Here's how the part is built. I have some questions about the finished solid (model axes, mm). A direction names the side the tool comes from. Round coordinates to 2 decimals unless told otherwise and drop trailing zeros. Write each loop counter-clockwise with the first axis right and the second up, starting at its lowest first coordinate (ties: lowest second). Pieces come first, ordered by that corner, then holes. Notation, with made-up numbers: (-37, -35.5) - (6, -35.5) arc R27 cw to (6, 2.5) - close; hole circle Ø8 at (79.5, 62.25). An arc over 180 degrees is marked (long way). One line per question, with ' | ' between items. Start each with the question number.
(1) Will these pins go through, and if not, where does the flat tip stop? pin 1 (1.5 mm diameter, centred on y = 41, z = 5, fed in from -X); pin 2 (5 mm diameter, centred on x = -3.5, y = 14.5, fed in from -Z); pin 3 (3 mm diameter, centred on y = 60, z = 5.5, fed in from +X).
(2) For faces 1 (the flat face through (-9.1, 33, 3)), 2 (the flat face through (6.1, 35, 3)), 3 (the flat face through (9.1, 34, 3)), which set-ups out of +Z, -Z, +X, -X, +Y, -Y let a thin tool reach every point of the face, with its end or its side?
(3) If I drill on L1, parallel to X at y = 9, z = 1.85; L2, parallel to Z at x = -13, y = 71; L3, parallel to Y at x = -13, z = 5.4, over which ranges is the centre line in solid material (lowest first)?
(4) Imagine slicing it at B-B (z = 3). Write out the boundary of the cut face in (x, y), plus the area to 3 significant figures.
(5) Imagine slicing it at A-A (y = 46.5). Write out the boundary of the cut face in (x, z).
(6) Imagine slicing it at C-C (x = 13.1). Write out the boundary of the cut face in (y, z).
(7) Imagine slicing it at D-D (x = -4). Write out the boundary of the cut face in (y, z).
(8) Thinking about a two-plate mould opening in Z: for faces 4 (the cylindrical face through (11.884, 71.479, 4.115)), 5 (the flat face through (17.1, 72, 3)), 6 (the flat face through (-6.3, 34.2, 6)), 7 (the flat face through (-6.3, 34.2, 0)), which applies, pulls with the +Z half, pulls with the -Z half, needs draft (parallel to the pull), parting line crosses it, or undercut?
from build123d import *

# Parameters (mm, degrees)
BOSS_EXTRUDE5_DEPTH = 6
SKETCH7_R           = 1.65
CUT_EXTRUDE2_DEPTH  = 3
FILLET1_R           = 1
FILLET2_R           = 1.5


with BuildPart() as part:
    # Sketch6 → Boss-Extrude5 (new body)
    with BuildSketch(Plane.XY):
        Polygon((-6.1, 0), (6.1, 0), (6.1, 73), (17.1, 73), (17.1, 70), (9.1, 70), (9.1, -5), (-9.1, -5), (-9.1, 70), (-17.1, 70), (-17.1, 73), (-6.1, 73), align=None)
    extrude(amount=BOSS_EXTRUDE5_DEPTH)

    # Sketch7 → Cut-Extrude2 (cut)
    with BuildSketch(Plane.XZ.offset(-70)):
        with Locations((-13.1, 3)):
            Circle(SKETCH7_R)
        with Locations((13.1, 3)):
            Circle(SKETCH7_R)
    extrude(amount=-CUT_EXTRUDE2_DEPTH, mode=Mode.SUBTRACT)

    # Fillet1
    fillet1_edges = [part.edges().sort_by_distance(p)[0] for p in [
        (6.1, 73, 3),
        (-6.1, 73, 3),
    ]]
    fillet(fillet1_edges, radius=FILLET1_R)

    # Fillet2
    fillet2_edges = [part.edges().sort_by_distance(p)[0] for p in [
        (9.1, -5, 3),
        (-9.1, -5, 3),
    ]]
    fillet(fillet2_edges, radius=FILLET2_R)


solid = part.part
Check sheet entries:
1) pin 1: x = -9.1 | pin 2: through | pin 3: x = 9.1
2) face 1: +Z, -Z, -X, -Y | face 2: +Z, -Z, +Y | face 3: +Z, -Z, +X, -Y
3) L1: -9.1 to -6.1, 6.1 to 9.1 | L2: 0 to 1.35, 4.65 to 6 | L3: 70 to 73
4) outline: (-17.1, 70) - (-14.75, 70) - (-14.75, 73) - (-17.1, 73) - close; (-11.45, 70) - (-9.1, 70) - (-9.1, -3.5) arc R1.5 ccw to (-7.6, -5) - (7.6, -5) arc R1.5 ccw to (9.1, -3.5) - (9.1, 70) - (11.45, 70) - (11.45, 73) - (7.1, 73) arc R1 ccw to (6.1, 72) - (6.1, 0) - (-6.1, 0) - (-6.1, 72) arc R1 ccw to (-7.1, 73) - (-11.45, 73) - close; (14.75, 70) - (17.1, 70) - (17.1, 73) - (14.75, 73) - close | area: 556 mm^2
5) outline: (-9.1, 0) - (-6.1, 0) - (-6.1, 6) - (-9.1, 6) - close; (6.1, 0) - (9.1, 0) - (9.1, 6) - (6.1, 6) - close
6) outline: (70, 0) - (73, 0) - (73, 1.35) - (70, 1.35) - close; (70, 4.65) - (73, 4.65) - (73, 6) - (70, 6) - close
7) outline: (-5, 0) - (0, 0) - (0, 6) - (-5, 6) - close
8) face 4: undercut | face 5: needs draft | face 6: pulls with the +Z half | face 7: pulls with the -Z half
